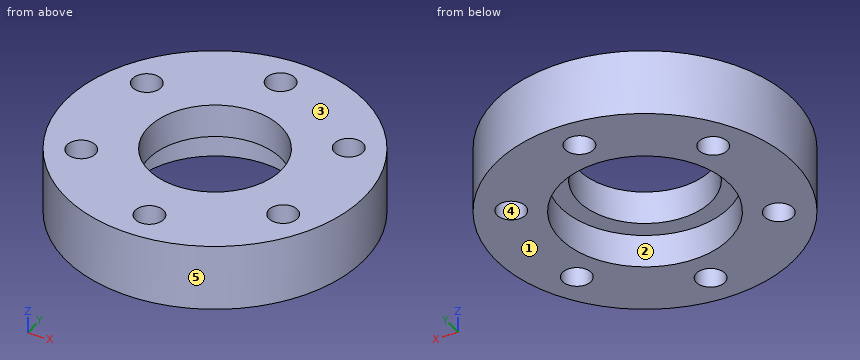
Autodesk Inventor part; units mm, degrees
ref_plane "YZ Plane" through (0, 0, 0) normal (1, 0, 0) x (0, 1, 0)
ref_plane "XZ Plane" through (0, 0, 0) normal (0, 1, 0) x (-1, 0, 0)
ref_plane "XY Plane" through (0, 0, 0) normal (0, 0, 1) x (1, 0, 0)
sketch "Sketch1" plane through (0, 0, 0) normal (0, 0, 1) x (1, 0, 0)
  circle A0 centre (0, 0) radius 22.5
  dimension "d0" = 45
extrude "Extrusion1" add sketch "Sketch1" along normal blind 10
sketch "Sketch4" plane through (0, 0, 10) normal (0, 0, 1) x (1, 0, 0)
  circle A0 centre (0, 0) radius 22.5
  circle A1 centre (0, 0) radius 17.5
  point P0 (0, 17.5)
  point P1 (-15.1554, 8.75)
  point P2 (-15.1554, -8.75)
  point P3 (0, -17.5)
  point P4 (15.1554, -8.75)
  point P5 (15.1554, 8.75)
  dimension "d18" = 35
  dimension "d21" = 360
hole "Hole3" at (0, 17.5, 10) at (-15.1554, 8.75, 10) at (-15.1554, -8.75, 10) at (0, -17.5, 10) at (15.1554, -8.75, 10) at (15.1554, 8.75, 10) direction (0, 0, -1) diameter 4.3 end through all
sketch "Sketch5" plane through (0, 0, 0) normal (0, 0, -1) x (-1, 0, 0)
  circle A0 centre (0, 0) radius 22.5
hole "Hole4" at (0, 0, 0) direction (0, 0, 1) diameter 25.5 depth 5
sketch "Sketch6" plane through (0, 0, 5) normal (0, 0, -1) x (-1, 0, 0)
  circle A0 centre (0, 0) radius 12.75
hole "Hole5" at (0, 0, 5) at (0, 0, 5) direction (0, 0, 1) diameter 20 end through all
properties part number "nylon clamp"
The listing builds one solid part. Answer for the finished solid, in the listing's coordinates (mm). Face numbers are marked on the shaded views. A direction names the side the tool comes from. Coordinates: 2 decimals unless noted, no trailing zeros. Loops run counter-clockwise (first coordinate to the right, second up) from the corner with the lowest first, then second, coordinate; pieces in that order, holes last. Notation, with made-up numbers: (-10, -8.5) -> (33, -8.5) arc R27 cw to (33, 27.5) -> close; hole circle Ø2 at (27.5, 61.5). An arc over 180 degrees is marked (long way). Return JSON: item names as keys, results as strings. Group by question number.
(1) A cutting plane is placed at C-C on z = 3.5. Write down the section's boundary in (x, y).
(2) A cutting plane is placed at D-D on y = 8.75. Write down the section's boundary in (x, z), and give its area (3 significant figures).
(3) Which of the six approach directions +Z, -Z, +X, -X, +Y, -Y give full straight-line access (tool end or side, diameter ignored) to the marked faces 1 and 2?
(4) Find the intervals of material crossed by probe 1 along Y at (x, z) = (0, 2.75); probe 2 along Y at (x, z) = (0, 7.6); probe 3 along X at (y, z) = (8.75, 4.25), in increasing order. Write a range as from..to.
(5) A cutting plane is placed at A-A on y = 0. Write down the section's boundary in (x, z), and give its area (4 significant figures).
(6) Given pin 1 Ø4 at (x, y) = (0, 17.5) entering from -Z; pin 2 Ø2 at (x, z) = (9.5, 1) entering from +Y; pin 3 Ø4 at (x, y) = (8, -3.5) entering from -Z; pin 4 Ø1.5 at (x, z) = (-4, 2.5) entering from +Y, each flat-ended and moving along its own axis, determine where each tip first touches the part or whether it passes through.
(7) Determine the mould class of the marked faces 3, 4 and 5 for opening direction X: released by +X, released by -X, zero draft, split by the parting line, or undercut.
(8) A cutting plane is placed at B-B on x = 0. Write down the section's boundary in (y, z).
The answers:
{
 "1": {"outline": "circle Ø45 at (0, 0); hole circle Ø4.3 at (-15.16, -8.75); hole circle Ø4.3 at (-15.16, 8.75); hole circle Ø25.5 at (0, 0); hole circle Ø4.3 at (0, -17.5); hole circle Ø4.3 at (0, 17.5); hole circle Ø4.3 at (15.16, -8.75); hole circle Ø4.3 at (15.16, 8.75)"},
 "2": {"outline": "(-20.73, 0) -> (-17.31, 0) -> (-17.31, 10) -> (-20.73, 10) -> close; (-13.01, 0) -> (-9.27, 0) -> (-9.27, 5) -> (-4.84, 5) -> (-4.84, 10) -> (-13.01, 10) -> close; (4.84, 5) -> (9.27, 5) -> (9.27, 0) -> (13.01, 0) -> (13.01, 10) -> (4.84, 10) -> close; (17.31, 0) -> (20.73, 0) -> (20.73, 10) -> (17.31, 10) -> close", "area": "187 mm^2"},
 "3": {"face 1": "-Z, +X, -X, +Y, -Y", "face 2": "-Z"},
 "4": {"probe 1": "y = -22.5..-19.65, -15.35..-12.75, 12.75..15.35, 19.65..22.5", "probe 2": "y = -22.5..-19.65, -15.35..-10, 10..15.35, 19.65..22.5", "probe 3": "x = -20.73..-17.31, -13.01..-9.27, 9.27..13.01, 17.31..20.73"},
 "5": {"outline": "(-22.5, 0) -> (-12.75, 0) -> (-12.75, 5) -> (-10, 5) -> (-10, 10) -> (-22.5, 10) -> close; (10, 5) -> (12.75, 5) -> (12.75, 0) -> (22.5, 0) -> (22.5, 10) -> (10, 10) -> close", "area": "222.5 mm^2"},
 "6": {"pin 1": "passes through", "pin 2": "stops at y = 20.83", "pin 3": "stops at z = 5", "pin 4": "stops at y = 22.26"},
 "7": {"face 3": "zero draft", "face 4": "undercut", "face 5": "split by the parting line"},
 "8": {"outline": "(-22.5, 0) -> (-19.65, 0) -> (-19.65, 10) -> (-22.5, 10) -> close; (-15.35, 0) -> (-12.75, 0) -> (-12.75, 5) -> (-10, 5) -> (-10, 10) -> (-15.35, 10) -> close; (10, 5) -> (12.75, 5) -> (12.75, 0) -> (15.35, 0) -> (15.35, 10) -> (10, 10) -> close; (19.65, 0) -> (22.5, 0) -> (22.5, 10) -> (19.65, 10) -> close"}
}
